The model under review builds one solid part; all positions refer to its coordinate system, in mm. Face numbers are marked on the shaded views. A direction names the side the tool comes from. Round coordinates to 2 decimals unless told otherwise and drop trailing zeros. Order: outer loops, then holes, each group sorted by start corner. A loop starts at its lowest first (then second) coordinate and runs counter-clockwise, first axis right, second up.
1) To check wall thickness, follow L1, parallel to Y at x = 20.5, z = 0; L2, parallel to X at y = 3.25, z = -4.75. State the ranges of each line that lie inside material, in increasing order.
2) Consider section A-A (x = 26). Give the boundary of the cut face in (y, z) (1 decimal).
3) Machinability: for the marked faces 1 and 2, which of the approach directions +Z, -Z, +X, -X, +Y, -Y give a long, thin tool a straight path to every point of the face, cutting with its end or side? Answer none if there is none.
4) Clearance check with flat-ended pins moving along their axes: P1, Ø2, axis at x = -1, z = 2.5, coming from the -Y side; P2, Ø4, axis at x = 8, z = -1, coming from the -Y side; P3, Ø1, axis at x = 15.5, z = 4.5, coming from the +Y side. State where each tip first meets the part, or that it passes through.
from build123d import *

# Parameters (mm, degrees)
SKETCH5_R           = 4.7625
BOSS_EXTRUDE3_DEPTH = 63.5
CHAMFER1_SIZE       = 1.190625
BOSS_EXTRUDE4_DEPTH = 5.953125
SKETCH8_OUTSIDE_W   = 274.906
SKETCH8_OUTSIDE_H   = 277.116
SKETCH8_OUTSIDE_R   = 7.14375
CUT_EXTRUDE3_DEPTH  = 70.453125
CUT_EXTRUDE3_TAPER  = 60


with BuildPart() as part:
    # Sketch5 → Boss-Extrude3 (new body)
    with BuildSketch(Plane(origin=(34.7265625, 0, 0), x_dir=(0, 0, -1), z_dir=(1, 0, 0))):
        Circle(SKETCH5_R)
    extrude(amount=-BOSS_EXTRUDE3_DEPTH)

    # Chamfer1
    chamfer1_edges = [part.edges().sort_by_distance(p)[0] for p in [
        (34.7265625, 0, 4.7625),
    ]]
    chamfer(chamfer1_edges, length=CHAMFER1_SIZE)

    # Sketch6 → Boss-Extrude4 (add)
    with BuildSketch(Plane.ZY.offset(28.7734375)):
        Polygon((7.14375, 4.124445986), (0, 8.248891971), (-7.14375, 4.124445986), (-7.14375, -4.124445986), (0, -8.248891971), (7.14375, -4.124445986), align=None)
    extrude(amount=BOSS_EXTRUDE4_DEPTH)

    # Sketch8 outside → Cut-Extrude3 (cut, through all)
    with BuildSketch(Plane.ZY.offset(34.7265625)):
        Rectangle(SKETCH8_OUTSIDE_W, SKETCH8_OUTSIDE_H)
        Circle(SKETCH8_OUTSIDE_R, mode=Mode.SUBTRACT)
    extrude(amount=-CUT_EXTRUDE3_DEPTH, taper=CUT_EXTRUDE3_TAPER, mode=Mode.SUBTRACT)


solid = part.part
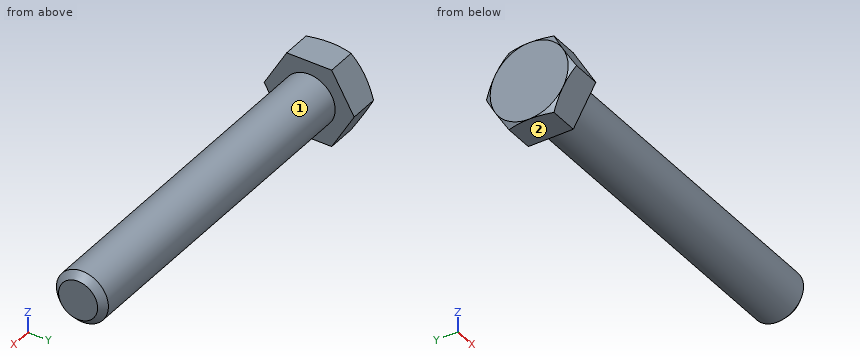
Answer below:
1. L1: y = -4.76 to 4.76
1. L2: x = -34.73 to -28.77
2. outline: circle Ø9.5 at (0, 0)
3. face 1: +X
3. face 2: -Z, +X, -X, +Y, -Y
4. P1: stops at y = -4.52
4. P2: stops at y = -4.76
4. P3: stops at y = 2.58
